Geometry: final body of the model. Coordinates: model frame, mm. A direction names the side the tool comes from. Coordinates: 2 decimals unless noted, no trailing zeros. Write each loop counter-clockwise with the first axis right and the second up, starting at its lowest first coordinate (ties: lowest second). Pieces come first, ordered by that corner, then holes. Notation, with made-up numbers: (86.25, 67.25) -> (92.25, 67.25) arc R21 ccw to (92.25, 76.25) -> close; hole circle Ø5 at (15.25, 72.5). An arc over 180 degrees is marked (long way). One line per item, written item: value.
```python
from build123d import *

# Parameters (mm, degrees)
CROQUIS1_W              = 30
CROQUIS1_H              = 68
SALIENTE_EXTRUIR1_DEPTH = 8
CROQUIS2_R              = 2.5
CORTAR_EXTRUIR1_DEPTH   = 47.043457733
CROQUIS3_R              = 2
CORTAR_EXTRUIR2_DEPTH   = 15
CROQUIS4_R              = 2.5
CORTAR_EXTRUIR3_DEPTH   = 39.013155617


with BuildPart() as part:
    # Croquis1 → Saliente-Extruir1 (new body)
    with BuildSketch(Plane.XY):
        Rectangle(CROQUIS1_W, CROQUIS1_H)
    extrude(amount=-SALIENTE_EXTRUIR1_DEPTH)

    # Croquis2 → Cortar-Extruir1 (cut, through all)
    with BuildSketch(Plane(origin=(15, 0, 0), x_dir=(0, 0, -1), z_dir=(1, 0, 0))):
        with Locations(Location((4, 30, 0), (0, 0, 90))):
            Circle(CROQUIS2_R)
    extrude(amount=-CORTAR_EXTRUIR1_DEPTH, mode=Mode.SUBTRACT)

    # Croquis3 → Cortar-Extruir2 (cut)
    with BuildSketch(Plane.XZ.offset(34)):
        with Locations(Location((-10, -4, 0), (0, 0, 270))):
            Circle(CROQUIS3_R)
        with Locations(Location((10, -4, 0), (0, 0, 270))):
            Circle(CROQUIS3_R)
    extrude(amount=-CORTAR_EXTRUIR2_DEPTH, mode=Mode.SUBTRACT)

    # Croquis4 → Cortar-Extruir3 (cut, through all)
    with BuildSketch(Plane.XY):
        with Locations((0, -12)):
            Circle(CROQUIS4_R)
    extrude(amount=-CORTAR_EXTRUIR3_DEPTH, mode=Mode.SUBTRACT)


solid = part.part
```
(1) Section C-C (x = 10). Return the cut outline in (y, z), then the cut area to 3 significant figures.
Responses:
outline: (-34, -8) -> (34, -8) -> (34, 0) -> (-34, 0) -> (-34, -2) -> (-19, -2) -> (-19, -6) -> (-34, -6) -> close; hole circle Ø5 at (30, -4)
area: 464 mm2
(2) Section A-A (z = -4). Return the cut outline in (x, y).
Responses:
outline: (-15, -34) -> (-12, -34) -> (-12, -19) -> (-8, -19) -> (-8, -34) -> (8, -34) -> (8, -19) -> (12, -19) -> (12, -34) -> (15, -34) -> (15, 27.5) -> (-15, 27.5) -> close; (-15, 32.5) -> (15, 32.5) -> (15, 34) -> (-15, 34) -> close; hole circle Ø5 at (0, -12)
(3) First-contact query: pin 1 (4 mm diameter, centred on y = 30, z = -4, fed in from +X). Flat tip, straight axial feed; report the tip coordinate or a pass-through.
Responses:
pin 1: passes through
(4) Section B-B (y = 30). Return the cut outline in (x, z).
Responses:
outline: (-15, -8) -> (15, -8) -> (15, -6.5) -> (-15, -6.5) -> close; (-15, -1.5) -> (15, -1.5) -> (15, 0) -> (-15, 0) -> close
(5) Section D-D (y = -12). Return the cut outline in (x, z).
Responses:
outline: (-15, -8) -> (-2.5, -8) -> (-2.5, 0) -> (-15, 0) -> close; (2.5, -8) -> (15, -8) -> (15, 0) -> (2.5, 0) -> close
(6) Reachability of faces 4 (the flat face through (0, 0, 0)), 5 (the flat face through (10, -19, -4)) from +Z, -Z, +X, -X, +Y, -Y: full face, straight path, thin tool, end or side. Return the list, or none.
Responses:
face 4: +Z, +X, -X, +Y, -Y
face 5: -Y
(7) Pull-direction query (X, two-part tool) for faces 1 (the cylindrical face through (-0.54, -14.44, -3.94)), 2 (the flat face through (-15, 0, -4)), 3 (the flat face through (0, -34, -4)); classes: released by +X, released by -X, zero draft, split by the parting line, or undercut.
Responses:
face 1: undercut
face 2: released by -X
face 3: zero draft
(8) Line query: line 1 (X direction, y = -27.5, z = -4); line 2 (Y direction, x = 2.25, z = -2.5); line 3 (Z direction, x = 8.5, y = 30). Output: solid intervals per line, ascending. Write a range as [from, to].
Responses:
line 1: x = [-15, -12], [-8, 8], [12, 15]
line 2: y = [-34, -13.09], [-10.91, 28], [32, 34]
line 3: z = [-8, -6.5], [-1.5, 0]
